Work out the finished part from the listing and answer in its coordinate system (mm). Face numbers are marked on the shaded views. Round coordinates to 2 decimals unless told otherwise and drop trailing zeros. Loops run counter-clockwise (first coordinate to the right, second up) from the corner with the lowest first, then second, coordinate; pieces in that order, holes last.
```python
from build123d import *

# Parameters (mm, degrees)
BOSS_EXTRUDE1_DEPTH = 30
SKETCH2_R           = 25
SKETCH2_R_2         = 12.5
CUT_EXTRUDE1_DEPTH  = 31


with BuildPart() as part:
    # Sketch1 → Boss-Extrude1 (new body)
    with BuildSketch(Plane(origin=(0, 0, 0), x_dir=(1, 0, 0), z_dir=(0, 1, 0))):
        with BuildLine():
            Line((115, -75), (-115, -75))
            ThreePointArc((-115, -75), (-122.071067812, -72.071067812), (-125, -65))
            Line((-125, -65), (-125, 65))
            ThreePointArc((-125, 65), (-122.071067812, 72.071067812), (-115, 75))
            Line((-115, 75), (115, 75))
            ThreePointArc((115, 75), (122.071067812, 72.071067812), (125, 65))
            Line((125, 65), (125, -65))
            ThreePointArc((125, -65), (122.071067812, -72.071067812), (115, -75))
        make_face()
    extrude(amount=BOSS_EXTRUDE1_DEPTH)

    # Sketch2 → Cut-Extrude1 (cut, through all)
    with BuildSketch(Plane(origin=(0, 30, 0), x_dir=(1, 0, 0), z_dir=(0, 1, 0))):
        with Locations((0, 25)):
            Circle(SKETCH2_R)
        with Locations((-95, 45)):
            Circle(SKETCH2_R_2)
        with Locations((95, 45)):
            Circle(SKETCH2_R_2)
        with Locations((95, -45)):
            Circle(SKETCH2_R_2)
        with Locations((-95, -45)):
            Circle(SKETCH2_R_2)
    extrude(amount=-CUT_EXTRUDE1_DEPTH, mode=Mode.SUBTRACT)


solid = part.part
```
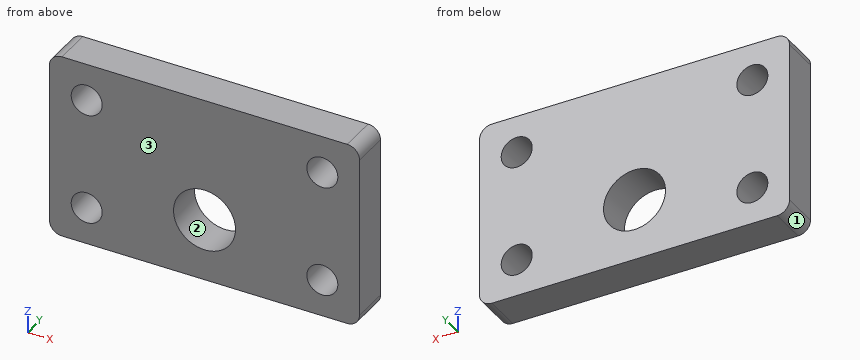
1. Determine the mould class of the marked faces 1, 2 and 3 for opening direction Z: +Z half, -Z half, draft (parallel to the pull), parting line (faces both ways), or undercut.
Answer key:
face 1: -Z half
face 2: undercut
face 3: draft
2. Consider probe 1 along Z at (x, y) = (-95, 10); probe 2 along X at (y, z) = (11, 45); probe 3 along Z at (x, y) = (105.5, 14.5). Determine where each line is inside the solid, lowest interval first.
Answer key:
probe 1: z = -75 to -57.5, -32.5 to 32.5, 57.5 to 75
probe 2: x = -125 to -107.5, -82.5 to 82.5, 107.5 to 125
probe 3: z = -75 to -51.78, -38.22 to 38.22, 51.78 to 75
3. Find section C-C (x = -95). Write down the section's boundary in (y, z), then the cut area to 3 significant figures.
Answer key:
outline: (0, -75) - (30, -75) - (30, -57.5) - (0, -57.5) - close; (0, -32.5) - (30, -32.5) - (30, 32.5) - (0, 32.5) - close; (0, 57.5) - (30, 57.5) - (30, 75) - (0, 75) - close
area: 3,000 mm2
4. Find section B-B (y = 20.25). Write down the section's boundary in (x, z), then the cut area to 3 significant figures.
Answer key:
outline: (-125, -65) arc R10 ccw to (-115, -75) - (115, -75) arc R10 ccw to (125, -65) - (125, 65) arc R10 ccw to (115, 75) - (-115, 75) arc R10 ccw to (-125, 65) - close; hole circle Ø25 at (-95, -45); hole circle Ø25 at (-95, 45); hole circle Ø50 at (0, -25); hole circle Ø25 at (95, -45); hole circle Ø25 at (95, 45)
area: 33,500 mm2
5. Find section A-A (z = -45). Write down the section's boundary in (x, y).
Answer key:
outline: (-125, 0) - (-107.5, 0) - (-107.5, 30) - (-125, 30) - close; (-82.5, 0) - (-15, 0) - (-15, 30) - (-82.5, 30) - close; (15, 0) - (82.5, 0) - (82.5, 30) - (15, 30) - close; (107.5, 0) - (125, 0) - (125, 30) - (107.5, 30) - close
6. Find section D-D (z = -25). Write down the section's boundary in (x, y).
Answer key:
outline: (-125, 0) - (-25, 0) - (-25, 30) - (-125, 30) - close; (25, 0) - (125, 0) - (125, 30) - (25, 30) - close
